Geometry check sheet. Reference: the model listing, model coordinates, mm. Face numbers are marked on the shaded views. A direction names the side the tool comes from. Coordinates: 2 decimals unless noted, no trailing zeros. Loops run counter-clockwise (first coordinate to the right, second up) from the corner with the lowest first, then second, coordinate; pieces in that order, holes last. Notation, with made-up numbers: M 27.5,40 L 41.5,40 A24 ccw 41.5,60 Z; hole C 67.5,15 d5. An arc over 180 degrees is marked long. One line per question, with ' | ' between items. Start each with the question number.
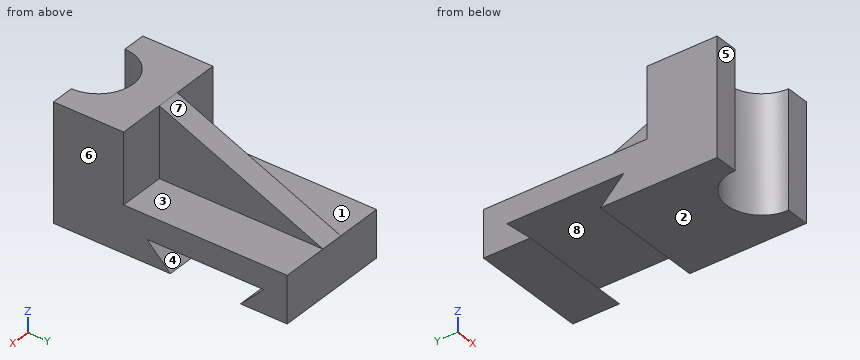
from build123d import *

# Parameters (mm, degrees)
PAD_DEPTH    = 25
SKETCH001_R  = 15
POCKET_DEPTH = 50.001
PAD001_DEPTH = 5


with BuildPart() as part:
    # Sketch → Pad (new body, symmetric)
    with BuildSketch(Plane.YZ):
        Polygon((0, 50), (0, 0), (50, 0), (40, 10), (90, 10), (80, 0), (100, 0), (100, 20), (30, 20), (30, 50), align=None)
    extrude(amount=PAD_DEPTH, both=True)

    # Sketch001 (on Face10 of Pad) → Pocket (cut, through all)
    with BuildSketch(Plane(origin=(0, 0, 50), x_dir=(0, -1, 0), z_dir=(0, 0, 1))):
        Circle(SKETCH001_R)
    extrude(amount=-POCKET_DEPTH, mode=Mode.SUBTRACT)

    # Sketch002 → Pad001 (join, symmetric)
    with BuildSketch(Plane.YZ):
        Polygon((30, 50), (30, 20), (100, 20), align=None)
    extrude(amount=PAD001_DEPTH, both=True)


solid = part.part
1. Sectioned sample at A-A (y = 61.5). Record the cut outline in (x, z), and give its area (3 significant figures).
2. Sectioned sample at D-D (z = 18.5). Record the cut outline in (x, y).
3. Thickness scan on line 1 (Y direction, x = -16.5, z = 22); line 2 (X direction, y = 5.5, z = 42); line 3 (Y direction, x = 2, z = 8). Record the ranges inside material, lowest first.
4. Draft check along Y on the marked faces 5, 6, 7 and 8. Enter one of: +Y half, -Y half, draft (parallel to the pull), parting line (faces both ways), or undercut.
5. Sectioned sample at B-B (x = 0). Record the cut outline in (y, z), and give its area (3 significant figures).
6. Depth check by flat-ended pin: pin 1 Ø5 at (x, z) = (5.5, 10.5) entering from -Y; pin 2 Ø15 at (y, z) = (51.5, 33) entering from -X; pin 3 Ø15 at (x, y) = (-6, 68) entering from -Z. Enter the tip coordinate at first touch or a pass-through.
7. Sectioned sample at C-C (y = 81). Record the cut outline in (x, z).
8. Tool access check on the marked faces 1, 2, 3 and 4. Record the directions out of +Z, -Z, +X, -X, +Y, -Y that give a thin tool (end or side, any length) a straight path to the whole face; none if there is none.
Result:
1) outline: M -25,10 L 25,10 L 25,20 L 5,20 L 5,36.5 L -5,36.5 L -5,20 L -25,20 Z | area: 665 mm2
2) outline: M -25,0 L -15,0 A15 cw 15,0 L 25,0 L 25,100 L -25,100 Z
3) line 1: y = 0 to 30 | line 2: x = -25 to -13.96, 13.96 to 25 | line 3: y = 14.87 to 42, 88 to 100
4) face 5: -Y half | face 6: draft | face 7: +Y half | face 8: undercut
5) outline: M 15,0 L 50,0 L 40,10 L 90,10 L 80,0 L 100,0 L 100,20 L 30,50 L 15,50 Z | area: 2,800 mm2
6) pin 1: stops at y = 12.69 | pin 2: stops at x = -5 | pin 3: stops at z = 10
7) outline: M -25,0 L 25,0 L 25,1 L -25,1 Z; M -25,10 L 25,10 L 25,20 L 5,20 L 5,28.14 L -5,28.14 L -5,20 L -25,20 Z
8) face 1: +Z, -X, +Y | face 2: -Z, +X, -X, +Y, -Y | face 3: +Z, +X, +Y | face 4: +X, -X
